Autodesk Inventor part; units mm, degrees
ref_plane "YZ Plane" through (0, 0, 0) normal (1, 0, 0) x (0, 1, 0)
ref_plane "XZ Plane" through (0, 0, 0) normal (0, 1, 0) x (-1, 0, 0)
ref_plane "XY Plane" through (0, 0, 0) normal (0, 0, 1) x (1, 0, 0)
sketch "Block1" plane through (0, 0, 0) normal (0, 0, 1) x (1, 0, 0)
  circle A0 centre (74.029, 24.2723) radius 1
  line L0 (49.279, 30.4723) -> (71.779, 30.4723)
  line L1 (71.779, 30.4723) -> (71.779, 18.0723)
  line L2 (71.779, 18.0723) -> (49.279, 18.0723)
  line L3 (49.279, 18.0723) -> (49.279, 30.4723)
  line L4 (49.279, 30.4723) -> (44.779, 30.4723)
  line L5 (44.779, 30.4723) -> (44.779, 18.0723)
  line L6 (44.779, 18.0723) -> (49.279, 18.0723)
  line L7 (49.279, 18.0723) -> (49.279, 30.4723)
  line L8 (71.779, 30.4723) -> (76.279, 30.4723)
  line L9 (76.279, 30.4723) -> (76.279, 18.0723)
  line L10 (76.279, 18.0723) -> (71.779, 18.0723)
  line L11 (71.779, 18.0723) -> (71.779, 30.4723)
  line L12 (44.779, 24.2723) -> (76.279, 24.2723) construction
  line L13 (47.029, 30.4723) -> (47.029, 18.0723) construction
  circle A1 centre (47.029, 24.2723) radius 1
  line L14 (74.029, 30.4723) -> (74.029, 18.0723) construction
  point P0 (60.979, 24.0984)
  dimension "d7" = 22.5
  dimension "d8" = 12.4
  dimension "d9" = 4.5
  dimension "d10" = 4.5
  dimension "d11" = 2
  dimension "d12" = 2
sketch "Sketch1" plane through (0, 0, 0) normal (0, 0, 1) x (1, 0, 0)
  line L0 (-92.7646, -8.503) -> (-89.7646, -8.503)
  line L1 (-89.7646, -8.503) -> (-89.7646, -11.753)
  line L2 (-89.7646, -11.753) -> (-92.7646, -11.753)
  line L3 (-92.7646, -11.753) -> (-92.7646, -8.503)
  line L4 (-92.7646, -21.6527) -> (-89.7646, -21.6527)
  line L5 (-89.7646, -21.6527) -> (-89.7646, -21.7527)
  line L6 (-89.7646, -21.7527) -> (-92.7646, -21.7527)
  line L7 (-92.7646, -21.7527) -> (-92.7646, -21.6527)
  line L8 (-51.3097, 56.2955) -> (-11.3097, 56.2955)
  line L9 (-11.3097, 56.2955) -> (-11.3097, 26.2955)
  line L10 (-11.3097, 26.2955) -> (-51.3097, 26.2955)
  line L11 (-51.3097, 26.2955) -> (-51.3097, 56.2955)
  line L12 (-51.3097, 41.2955) -> (-11.3097, 41.2955) construction
  line L13 (-21.3097, 48.2955) -> (-18.0597, 48.2955)
  line L14 (-18.0597, 48.2955) -> (-18.0597, 34.2955)
  line L15 (-18.0597, 34.2955) -> (-21.3097, 34.2955)
  line L16 (-21.3097, 34.2955) -> (-21.3097, 48.2955)
  line L17 (-21.3097, 41.2955) -> (-18.0597, 41.2955) construction
  line L18 (-11.3097, 66.2955) -> (18.6903, 66.2955)
  line L19 (18.6903, 66.2955) -> (18.6903, 16.2955)
  line L20 (18.6903, 16.2955) -> (-11.3097, 16.2955)
  line L21 (-11.3097, 16.2955) -> (-11.3097, 66.2955)
  line L22 (-11.3097, 41.2955) -> (18.6903, 41.2955) construction
  line L23 (-38.3097, 56.2955) -> (-38.3097, 26.2955) construction
  arc A0 (-38.3097, 56.2955) -> (-38.3097, 26.2955) centre (-36.1559, 41.2955) ccw
  circle A1 centre (9.1348, 41.2955) radius 25
  arc A2 (-31.9326, 56.2955) -> (-1.361, 63.9855) centre (-33.7351, 128.0749) ccw
  line L24 (-31.9326, 56.2955) -> (-31.9326, 53.1229)
  line L25 (-31.9326, 53.1229) -> (-1.361, 53.1229)
  line L26 (-1.361, 53.1229) -> (-1.361, 63.9855)
  arc A3 (-1.361, 18.6054) -> (-31.9326, 26.2955) centre (-33.7351, -45.4839) ccw
  line L27 (-31.9326, 26.2955) -> (-31.9326, 29.468)
  line L28 (-31.9326, 29.468) -> (-1.361, 29.468)
  line L29 (-1.361, 29.468) -> (-1.361, 18.6054)
  point P0 (0, 0)
  dimension "d0" = 3
  dimension "mat" = 3.25
  dimension "d2" = 3
  dimension "d3" = 0.1
  dimension "d23" = 40
  dimension "d24" = 30
  dimension "d29" = 3.25
  dimension "d30" = 14
  dimension "d31" = 30
  dimension "d38" = 30
  dimension "d39" = 50
  dimension "d42" = 13
  dimension "d43" = 50
extrude "Extrusion6" add sketch "Sketch1" along normal blind 3.25 contours L8 L24 L25 A1 L28 L27 L10 A0 | L8 L9 A1 L25 L24 | L27 L28 A1 L9 L10 | A1 A2 L26 L25 L9 | L9 L25 A1 | A1 A2 | L25 L9 L28 A1 | L25 L26 A1 L19 L29 L28 L9 | L28 L9 A1 | L9 L28 L29 A3 A1 | A3 A1 | A1 L19
extrude "Extrusion7" add sketch "Sketch1" along normal blind 3.25 contours A2 L21 L8 | L8 L9 A1 L25 L24 | L21 A2 A1 L9 | A1 A2 L26 L25 L9 | L9 L25 A1
extrude "Extrusion8" add sketch "Sketch1" along normal blind 3.25 contours L27 L28 A1 L9 L10 | L10 L21 A3 | L9 A1 A3 L21 | L28 L9 A1 | L9 L28 L29 A3 A1
equation "\"d29\" = mat"
equation "\"d44\" = mat"
equation "\"d46\" = mat"
equation "\"d48\" = mat"
properties part number "arm-servo"
Design review of the part built by this model. Coordinates are the model's own, in mm. A direction names the side the tool comes from. Give positions to 0.01 mm unless a question says otherwise; leave off trailing zeros. Order: outer loops, then holes, each group sorted by start corner. A loop starts at its lowest first (then second) coordinate and runs counter-clockwise, first axis right, second up.
1. Tool access review of faces 4 (the flat face through (0, 42, 3.25)), 5 (the flat face through (-35, 56.296, 2)), 6 (the flat face through (-18.06, 41, 2)): name each direction out of +Z, -Z, +X, -X, +Y, -Y from which nothing blocks a thin tool from reaching the whole face with its end or side.
Solution:
face 4: +Z, +X, -X, +Y, -Y
face 5: +Z, -Z, -X, +Y
face 6: +Z, -Z
2. Add section B-B, the plane z = 0.75. State the section outline as (x, y) points.
Solution:
outline: (-38.31, 26.3) - (-31.93, 26.3) arc R71.8 cw to (-2.51, 19.17) arc R25 ccw (long way) to (-2.51, 63.42) arc R71.8 cw to (-31.93, 56.3) - (-38.31, 56.3) arc R15.15 ccw to start; hole (-21.31, 34.3) - (-18.06, 34.3) - (-18.06, 48.3) - (-21.31, 48.3) - close
3. To check wall thickness, follow L1, parallel to X at y = 35, z = 2.1; L2, parallel to X at y = 35.5, z = 2.8; L3, parallel to Y at x = 9, z = 1.85. State the ranges of each line that lie inside material, in increasing order.
Solution:
L1: x = -49.94 to -21.31, -18.06 to 33.33
L2: x = -50.16 to -21.31, -18.06 to 33.45
L3: y = 16.3 to 66.3
4. Add section C-C, the plane y = 47. State the section outline as (x, z) points, then the cut area to 3 significant figures.
Solution:
outline: (-50.2, 0) - (-21.31, 0) - (-21.31, 3.25) - (-50.2, 3.25) - close; (-18.06, 0) - (33.48, 0) - (33.48, 3.25) - (-18.06, 3.25) - close
area: 261 mm2
5. Add section D-D, the plane y = 28.5. State the section outline as (x, z) points.
Solution:
outline: (-44.27, 0) - (30.61, 0) - (30.61, 3.25) - (-44.27, 3.25) - close
6. Mouldability with a two-part tool opening along Y and no side actions: class faces 1 (the flat face through (0, 42, 0)), 2 (the flat face through (-20, 48.296, 2)), 3 (the flat face through (-35, 26.296, 2)) as +Y half, -Y half, draft (parallel to the pull), parting line (faces both ways), or undercut.
Solution:
face 1: draft
face 2: undercut
face 3: -Y half
7. Add section A-A, the plane x = -20. State the section outline as (y, z) points.
Solution:
outline: (24.99, 0) - (34.3, 0) - (34.3, 3.25) - (24.99, 3.25) - close; (48.3, 0) - (57.6, 0) - (57.6, 3.25) - (48.3, 3.25) - close
8. For pin 1 Ø1 at (x, z) = (-20, 1) entering from +Y, flat-tipped, find the tip position at first contact; note if it passes through.
Solution:
pin 1: stops at y = 57.7
